For this review, take the finished solid that the model builds, in its own axes (mm). A direction names the side the tool comes from. Round coordinates to 2 decimals unless told otherwise and drop trailing zeros. Order: outer loops, then holes, each group sorted by start corner. A loop starts at its lowest first (then second) coordinate and runs counter-clockwise, first axis right, second up.
```python
from build123d import *

# Parameters (mm, degrees)
EXTRUDE_2_DEPTH = 1
SKETCH_1_4_W    = 2.7
SKETCH_1_4_H    = 2.2
SKETCH_1_4_R    = 1.25
EXTRUDE_3_DEPTH = 3
FILLET_1_R      = 0.5
FILLET_2_R      = 2


with BuildPart() as part:
    # 草图1 → 凸台-拉伸2 (new body)
    with BuildSketch(Plane(origin=(0, 0, 0), x_dir=(1, 0, 0), z_dir=(0, 1, 0))):
        with BuildLine():
            ThreePointArc((-3, 12.25), (0, 15.25), (3, 12.25))
            Line((3, 12.25), (7, 12.25))
            ThreePointArc((7, 12.25), (0, 19.25), (-7, 12.25))
            Line((-7, 12.25), (-3, 12.25))
        make_face()
        with BuildLine():
            ThreePointArc((3, 12.25), (2.121320344, 10.128679656), (0, 9.25))
            Line((0, 9.25), (0, 5.25))
            ThreePointArc((0, 5.25), (4.949747468, 7.300252532), (7, 12.25))
            Line((7, 12.25), (3, 12.25))
        make_face()
        with BuildLine():
            Line((0, 5.25), (0, 9.25))
            ThreePointArc((0, 9.25), (-2.121320344, 10.128679656), (-3, 12.25))
            Line((-3, 12.25), (-7, 12.25))
            ThreePointArc((-7, 12.25), (-4.949747468, 7.300252532), (0, 5.25))
        make_face()
    extrude(amount=EXTRUDE_2_DEPTH)

    # 草图1<4> → 凸台-拉伸3 (add)
    with BuildSketch(Plane(origin=(0, 0, 0), x_dir=(1, 0, 0), z_dir=(0, 1, 0))):
        with BuildLine():
            ThreePointArc((7, 12.25), (4.949747468, 7.300252532), (0, 5.25))
            ThreePointArc((0, 5.25), (-4.949747468, 7.300252532), (-7, 12.25))
            Line((-7, 12.25), (-7, -12.25))
            Line((-7, -12.25), (7, -12.25))
            Line((7, -12.25), (7, 12.25))
        make_face()
        with Locations((-3.75, -9.170716156)):
            Rectangle(SKETCH_1_4_W, SKETCH_1_4_H, mode=Mode.SUBTRACT)
        with Locations((0, -9.25)):
            Circle(SKETCH_1_4_R, mode=Mode.SUBTRACT)
        with Locations((3.75, -9.170716156)):
            Rectangle(SKETCH_1_4_W, SKETCH_1_4_H, mode=Mode.SUBTRACT)
        with BuildLine():
            ThreePointArc((1, 2.25), (-0.707106781, 1.542893219), (0, 3.25))
            ThreePointArc((0, 3.25), (0.707106781, 2.957106781), (1, 2.25))
        make_face(mode=Mode.SUBTRACT)
    extrude(amount=EXTRUDE_3_DEPTH)

    # 圆角1
    fillet_1_edges = [part.edges().sort_by_distance(p)[0] for p in [
        (7, 2, -12.25),
        (-7, 2, -12.25),
    ]]
    fillet(fillet_1_edges, radius=FILLET_1_R)

    # 圆角2
    fillet_2_edges = [part.edges().sort_by_distance(p)[0] for p in [
        (7, 1.5, 12.25),
        (-7, 1.5, 12.25),
    ]]
    fillet(fillet_2_edges, radius=FILLET_2_R)


solid = part.part
```
Q1. Clearance check with flat-ended pins moving along their axes: pin 1 (1.3 mm diameter, centred on x = 3.5, y = 2, fed in from -Z); pin 2 (0.8 mm diameter, centred on x = -4, y = 1.5, fed in from -Z); pin 3 (4 mm diameter, centred on x = -1.5, z = -13.5, fed in from +Y); pin 4 (1.8 mm diameter, centred on x = 0, z = -2.25, fed in from +Y). State where each tip first meets the part, or that it passes through.
Q2. Take a section at D-D, the plane z = -7.5. State the section outline as (x, y) points, plus the area to 3 significant figures.
Q3. Wall thickness on line 1 (Z direction, x = 0, y = 1.7); line 2 (Z direction, x = 0, y = 0.7); line 3 (X direction, y = 0.7, z = 9.25): over which ranges is each line inside the solid? List them lowest first.
Q4. Mouldability with a two-part tool opening along Z and no side actions: class faces 1 (the face through (0, 1, 12.25)), 2 (the face through (0.15, 0.49, -19.25)), 3 (the face through (-5.1, 1, 9)) as +Z half, -Z half, draft (parallel to the pull), parting line (faces both ways), or undercut.
Q5. Take a section at C-C, the plane x = -2. State the section outline as (y, z) points.
Q6. Take a section at B-B, the plane y = 1.6. State the section outline as (x, z) points, plus the area to 3 significant figures.
Q7. Tool access review of faces 4 (the face through (0, 3, 1)), 5 (the face through (5.1, 1, 9)), 6 (the face through (-6.6, 2, -9)): name each direction out of +Z, -Z, +X, -X, +Y, -Y from which nothing blocks a thin tool from reaching the whole face with its end or side.
Q8. Take a section at A-A, the plane z = 9.25. State the section outline as (x, y) points.
Working result:
1. pin 1: stops at z = -6.61
1. pin 2: stops at z = -6.81
1. pin 3: stops at y = 1
1. pin 4: passes through
2. outline: (-7, 0) - (7, 0) - (7, 3) - (5.14, 3) - (5.14, 1) - (-5.14, 1) - (-5.14, 3) - (-7, 3) - close
2. area: 21.4 mm2
3. line 1: z = -5.25 to -3.25, -1.25 to 8, 10.5 to 12.25
3. line 2: z = -19.25 to -15.25, -9.25 to -3.25, -1.25 to 8, 10.5 to 12.25
3. line 3: x = -7 to -5.1, -2.4 to -1.25, 1.25 to 2.4, 5.1 to 7
4. face 1: +Z half
4. face 2: -Z half
4. face 3: undercut
5. outline: (0, -18.96) - (1, -18.96) - (1, -14.49) - (0, -14.49) - close; (0, -10.01) - (1, -10.01) - (1, -5.54) - (3, -5.54) - (3, 12.25) - (0, 12.25) - close
6. outline: (-7, -8.51) arc R0.5 ccw to (-6.07, -8.76) arc R7 cw to (6.07, -8.76) arc R0.5 ccw to (7, -8.51) - (7, 10.25) arc R2 ccw to (5, 12.25) - (-5, 12.25) arc R2 ccw to (-7, 10.25) - close; hole (-5.1, 8.07) - (-2.4, 8.07) - (-2.4, 10.27) - (-5.1, 10.27) - close; hole circle Ø2.5 at (0, 9.25); hole circle Ø2 at (0, -2.25); hole (2.4, 8.07) - (5.1, 8.07) - (5.1, 10.27) - (2.4, 10.27) - close
6. area: 243 mm2
7. face 4: +Z, -Z, +X, -X, +Y
7. face 5: +Y, -Y
7. face 6: -Z, +Y
8. outline: (-7, 0) - (-5.1, 0) - (-5.1, 3) - (-7, 3) - close; (-2.4, 0) - (-1.25, 0) - (-1.25, 3) - (-2.4, 3) - close; (1.25, 0) - (2.4, 0) - (2.4, 3) - (1.25, 3) - close; (5.1, 0) - (7, 0) - (7, 3) - (5.1, 3) - close
